Input: part model. Units: mm. Frame: model coordinates. A direction names the side the tool comes from. Coordinates: 2 decimals unless noted, no trailing zeros. Loops run counter-clockwise (first coordinate to the right, second up) from the corner with the lowest first, then second, coordinate; pieces in that order, holes last.
Item 1: Contact query for flat-ended pins moving along their axis: P1, Ø7.5, axis at x = 1, z = 422.5, coming from the -Y side; P2, Ø4, axis at x = -8, y = -10.5, coming from the -Z side; P3, Ø12, axis at x = 7.5, z = 171.5, coming from the +Y side. Output: stop coordinate, or through.
Item 2: Section A-A on x = -6.5. Return loops of the section in (y, z).
Item 3: Ray query, line 1 along Z through (x, y) = (-16, -12); line 2 along Z through (x, y) = (-10.5, 7); line 3 along Y through (x, z) = (10, 120.5). Return the intervals inside material, ascending.
Item 4: Reachability of faces 4 (the flat face through (20, -20, -11)), 5 (the flat face through (-15, 0, 25)), 6 (the cylindrical face through (11.923, 3.755, 212.34)), 7 (the flat face through (14, 0, 405)), 8 (the flat face through (0, 12.5, 13)) from +Z, -Z, +X, -X, +Y, -Y: full face, straight path, thin tool, end or side. Return the list, or none.
Item 5: Section B-B on z = 347.5. Return loops of the section in (x, y), and give its area (3 significant figures).
Item 6: Pull-direction query (Y, two-part tool) for faces 1 (the flat face through (-20, 0, 418)), 2 (the cylindrical face through (-3.755, -15.403, 13.959)), 3 (the flat face through (0, 12.5, 418)); classes: released by +Y, released by -Y, zero draft, split by the parting line, or undercut.
```python
from build123d import *

# Parameters (mm, degrees)
ESQUISSE3_R                  = 12.5
BOSS_EXTRU_1_DEPTH           = 430
BOSS_EXTRU_2_DEPTH           = 20
BOSS_EXTRU_2_DEPTH_BACK      = 20
ESQUISSE4_W                  = 25
ESQUISSE4_H                  = 25
ENL_V_MAT_EXTRU_1_DEPTH      = 433.037324776
ENL_V_MAT_EXTRU_1_DEPTH_BACK = 433.037324776
ESQUISSE9_R                  = 12.5
BOSS_EXTRU_3_DEPTH           = 20
BOSS_EXTRU_4_DEPTH           = 40
ENL_V_MAT_EXTRU_2_DEPTH      = 434.766210072
ENL_V_MAT_EXTRU_2_DEPTH_BACK = 434.766210072
ESQUISSE12_R                 = 12.5
BOSS_EXTRU_5_DEPTH           = 70


with BuildPart() as part:
    # Esquisse3 → Boss.-Extru.1 (new body)
    with BuildSketch(Plane.XY):
        Circle(ESQUISSE3_R)
    extrude(amount=BOSS_EXTRU_1_DEPTH)

    # Esquisse4 → Boss.-Extru.2 (add, two sides: drawn at the far end of the back side and taken through both)
    with BuildSketch(Plane(origin=(0, 0, 0), x_dir=(0, 0, -1), z_dir=(1, 0, 0)).offset(-BOSS_EXTRU_2_DEPTH_BACK)):
        with Locations((-417.5, 0)):
            Rectangle(ESQUISSE4_W, ESQUISSE4_H)
        with Locations((-12.5, 0)):
            Rectangle(ESQUISSE4_W, ESQUISSE4_H)
    extrude(amount=BOSS_EXTRU_2_DEPTH + BOSS_EXTRU_2_DEPTH_BACK)

    # Esquisse8 → Enlèv. mat.-Extru.1 (cut, two sides: drawn at the far end of the back side and taken through both)
    with BuildSketch(Plane(origin=(20, 0, 0), x_dir=(0, 0, -1), z_dir=(1, 0, 0)).offset(-ENL_V_MAT_EXTRU_1_DEPTH_BACK)):
        Polygon((0, 12.5), (-25, -12.5), (0, -12.5), align=None)
    extrude(amount=ENL_V_MAT_EXTRU_1_DEPTH + ENL_V_MAT_EXTRU_1_DEPTH_BACK, mode=Mode.SUBTRACT)

    # Esquisse9 → Boss.-Extru.3 (add)
    with BuildSketch(Plane(origin=(0, 6.25, 6.25), x_dir=(-1, 0, 0), z_dir=(0, -0.7071067811865462, -0.707106781186549))):
        with Locations(Location((0, -8.838834765, 0), (0, 0, 270))):
            Circle(ESQUISSE9_R)
    extrude(amount=BOSS_EXTRU_3_DEPTH)

    # Esquisse10 → Boss.-Extru.4 (add)
    with BuildSketch(Plane(origin=(20, 0, 0), x_dir=(0, 0, -1), z_dir=(1, 0, 0))):
        Polygon((-7.196699141, -22.980970389), (10.480970389, -5.303300859), (28.158639918, -22.980970389), (10.480970389, -40.658639918), align=None)
    extrude(amount=-BOSS_EXTRU_4_DEPTH)

    # Esquisse11 → Enlèv. mat.-Extru.2 (cut, two sides: drawn at the far end of the back side and taken through both)
    with BuildSketch(Plane(origin=(20, 0, 0), x_dir=(0, 0, -1), z_dir=(1, 0, 0)).offset(-ENL_V_MAT_EXTRU_2_DEPTH_BACK)):
        Polygon((28.158639918, -22.980970389), (0.274763127, -30.452432657), (10.480970389, -40.658639918), align=None)
    extrude(amount=ENL_V_MAT_EXTRU_2_DEPTH + ENL_V_MAT_EXTRU_2_DEPTH_BACK, mode=Mode.SUBTRACT)

    # Esquisse12 → Boss.-Extru.5 (add)
    with BuildSketch(Plane(origin=(0, -28.481197254, -7.631513804), x_dir=(1, 0, 0), z_dir=(0, -0.9659258262890676, -0.2588190451025233))):
        with Locations(Location((0, -6.817487989, 0), (0, 0, 90))):
            Circle(ESQUISSE12_R)
    extrude(amount=BOSS_EXTRU_5_DEPTH)


solid = part.part
```
Results found:
1. P1: stops at y = -12.5
1. P2: stops at z = -17.68
1. P3: stops at y = 12.41
2. outline: (-97.09, -22.02) - (-91.57, -42.65) - (-23.95, -24.53) - (-22.98, -28.16) - (-5.3, -10.48) - (-6.59, -9.19) - (7.55, 4.95) - (12.5, 0) - (12.5, 25) - (10.68, 25) - (10.68, 405) - (12.5, 405) - (12.5, 430) - (-12.5, 430) - (-12.5, 405) - (-10.68, 405) - (-10.68, 25) - (-12.5, 25) - (-7.55, 20.05) - (-21.69, 5.91) - (-22.98, 7.2) - (-30.45, -0.27) - (-29.48, -3.9) - close
3. line 1: z = -17.18 to -3.78, 24.5 to 25, 405 to 430
3. line 2: z = 5.5 to 25, 405 to 430
3. line 3: y = -7.5 to 7.5
4. face 4: +Z, -Z, +X, +Y, -Y
4. face 5: -X
4. face 6: none
4. face 7: +X
4. face 8: +Z, -Z, +X, -X, +Y
5. outline: circle Ø25 at (0, 0)
5. area: 491 mm2
6. face 1: zero draft
6. face 2: undercut
6. face 3: released by +Y
